from build123d import *

# Parameters (mm, degrees)
SKETCH1_W           = 40
SKETCH1_H           = 30
BOSS_EXTRUDE1_DEPTH = 20
FILLET1_R           = 5
SKETCH2_R           = 5
CUT_EXTRUDE1_DEPTH  = 10
SKETCH3_W           = 25
SKETCH3_H           = 25
CUT_EXTRUDE2_DEPTH  = 10


with BuildPart() as part:
    # Sketch1 → Boss-Extrude1 (new body)
    with BuildSketch(Plane.XY):
        Rectangle(SKETCH1_W, SKETCH1_H)
    extrude(amount=BOSS_EXTRUDE1_DEPTH)

    # Fillet1
    fillet1_edges = [part.edges().sort_by_distance(p)[0] for p in [
        (20, -15, 10),
        (-20, -15, 10),
        (-20, 15, 10),
        (20, 15, 10),
    ]]
    fillet(fillet1_edges, radius=FILLET1_R)

    # Sketch2 → Cut-Extrude1 (cut)
    with BuildSketch(Plane(origin=(0, 0, 0), x_dir=(-1, 0, 0), z_dir=(0, 0, -1))):
        with Locations((-8.75, 0)):
            Circle(SKETCH2_R)
        with Locations((8.75, 0)):
            Circle(SKETCH2_R)
    extrude(amount=-CUT_EXTRUDE1_DEPTH, mode=Mode.SUBTRACT)

    # Sketch3 → Cut-Extrude2 (cut)
    with BuildSketch(Plane.XY.offset(20)):
        with Locations((0, -2.5)):
            Rectangle(SKETCH3_W, SKETCH3_H)
    extrude(amount=-CUT_EXTRUDE2_DEPTH, mode=Mode.SUBTRACT)


solid = part.part
Read the model definition and answer for the solid it produces. Units are mm, in the model's axes. A direction names the side the tool comes from. Coordinates: 2 decimals unless noted, no trailing zeros. Order: outer loops, then holes, each group sorted by start corner. A loop starts at its lowest first (then second) coordinate and runs counter-clockwise, first axis right, second up. Notation, with made-up numbers: (41, 85.25) -> (55, 85.25) arc R24 cw to (55, 110.25) -> close; hole circle Ø5 at (-30.5, 19.25). An arc over 180 degrees is marked (long way). Answer as a JSON object with one key per item and string values.
1) A cutting plane is placed at D-D, the plane y = 4. Determine the outline of the cut face in (x, z), plus the area to 3 significant figures.
Model answer:
{"outline": "(-20, 0) -> (-11.75, 0) -> (-11.75, 10) -> (-12.5, 10) -> (-12.5, 20) -> (-20, 20) -> close; (-5.75, 0) -> (5.75, 0) -> (5.75, 10) -> (-5.75, 10) -> close; (11.75, 0) -> (20, 0) -> (20, 20) -> (12.5, 20) -> (12.5, 10) -> (11.75, 10) -> close", "area": "430 mm²"}
2) A cutting plane is placed at C-C, the plane z = 18.5. Determine the outline of the cut face in (x, y).
Model answer:
{"outline": "(-20, -10) arc R5 ccw to (-15, -15) -> (-12.5, -15) -> (-12.5, 10) -> (12.5, 10) -> (12.5, -15) -> (15, -15) arc R5 ccw to (20, -10) -> (20, 10) arc R5 ccw to (15, 15) -> (-15, 15) arc R5 ccw to (-20, 10) -> close"}
3) Consider line 1 along X through (y, z) = (0, 6.5); line 2 along Y through (x, z) = (-8.75, 5); line 3 along X through (y, z) = (3, 4.25). Determine where each line is inside the solid, lowest interval first. Write a range as from..to.
Model answer:
{"line 1": "x = -20..-13.75, -3.75..3.75, 13.75..20", "line 2": "y = -15..-5, 5..15", "line 3": "x = -20..-12.75, -4.75..4.75, 12.75..20"}
4) Each of these flat-tipped pins is pushed along its axis until it touches: pin 1 (2 mm diameter, centred on x = -9, y = -9.5, fed in from +Z); pin 2 (3 mm diameter, centred on x = -3.5, z = 16.5, fed in from -Y); pin 3 (1 mm diameter, centred on x = 13, y = -1, fed in from -Z). Where does it stop, or does it pass through?
Model answer:
{"pin 1": "stops at z = 10", "pin 2": "stops at y = 10", "pin 3": "stops at z = 10"}
5) The mould has two halves that part along Y. Classify faces 4 (the face through (12.5, -3, 15)), 5 (the face through (13, 0, 10)), 6 (the face through (18, -14, 10)): released by +Y, released by -Y, zero draft, split by the parting line, or undercut.
Model answer:
{"face 4": "zero draft", "face 5": "undercut", "face 6": "released by -Y"}
6) A cutting plane is placed at B-B, the plane x = -8.75. Determine the outline of the cut face in (y, z), plus the area to 3 significant figures.
Model answer:
{"outline": "(-15, 0) -> (-5, 0) -> (-5, 10) -> (-15, 10) -> close; (5, 0) -> (15, 0) -> (15, 20) -> (10, 20) -> (10, 10) -> (5, 10) -> close", "area": "250 mm²"}
7) A cutting plane is placed at A-A, the plane y = 0. Determine the outline of the cut face in (x, z), plus the area to 3 significant figures.
Model answer:
{"outline": "(-20, 0) -> (-13.75, 0) -> (-13.75, 10) -> (-12.5, 10) -> (-12.5, 20) -> (-20, 20) -> close; (-3.75, 0) -> (3.75, 0) -> (3.75, 10) -> (-3.75, 10) -> close; (12.5, 10) -> (13.75, 10) -> (13.75, 0) -> (20, 0) -> (20, 20) -> (12.5, 20) -> close", "area": "350 mm²"}
8) A tool of negligible diameter and unlimited length cuts with its end or side. For faces 1 (the face through (3.98, 1.5, 4.93)), 2 (the face through (0, 10, 15)), 3 (the face through (19, 13, 10)), from which of +Z, -Z, +X, -X, +Y, -Y can it reach the whole face along a straight path? Write none if from no direction.
Model answer:
{"face 1": "-Z", "face 2": "+Z, -Y", "face 3": "+Z, -Z, +X, +Y"}
